```python
from build123d import *

# Parameters (mm, degrees)
SKETCH2_W             = 470
SKETCH2_H             = 317
BOSS_EXTRUDE1_DEPTH   = 5
SKETCH3_R             = 4.05
CUT_EXTRUDE1_DEPTH    = 10
SKETCH4_R             = 9
CUT_EXTRUDE2_DEPTH    = 11
M5X0_8_TAPPED_HOLE1_D = 4.2
SKETCH7_R             = 19.1
CUT_EXTRUDE5_DEPTH    = 2
M5X0_8_TAPPED_HOLE2_D = 4.2
SKETCH19_R            = 15
CUT_EXTRUDE10_DEPTH   = 9
SKETCH20_W            = 14
SKETCH20_H            = 30
CUT_EXTRUDE11_DEPTH   = 2
M3X0_5_TAPPED_HOLE2_D = 2.5
SKETCH23_W            = 14
SKETCH23_H            = 13.5
CUT_EXTRUDE13_DEPTH   = 9
CUT_EXTRUDE14_DEPTH   = 11
FILLET1_R             = 3
FILLET2_R             = 2.5
SKETCH27_R            = 4.05
CUT_EXTRUDE15_DEPTH   = 11
CUT_EXTRUDE16_DEPTH   = 11
CUT_EXTRUDE17_DEPTH   = 11


with BuildPart() as part:
    # Sketch2 → Boss-Extrude1 (new body, symmetric)
    with BuildSketch(Plane.XY):
        Rectangle(SKETCH2_W, SKETCH2_H)
    extrude(amount=BOSS_EXTRUDE1_DEPTH, both=True)

    # Sketch3 → Cut-Extrude1 (cut)
    with BuildSketch(Plane.XY.offset(5)):
        with Locations((-215, -83.5)):
            Circle(SKETCH3_R)
        with Locations((-215, -143.5)):
            Circle(SKETCH3_R)
        with Locations((215, -143.5)):
            Circle(SKETCH3_R)
        with Locations((-62.5, 133.34)):
            Circle(SKETCH3_R)
        with Locations((215, 138.5)):
            Circle(SKETCH3_R)
    extrude(amount=-CUT_EXTRUDE1_DEPTH, mode=Mode.SUBTRACT)

    # Sketch4 → Cut-Extrude2 (cut, through all)
    with BuildSketch(Plane.XY.offset(5)):
        with Locations((112.65, 121)):
            Circle(SKETCH4_R)
        with Locations((112.65, 26.5)):
            Circle(SKETCH4_R)
    extrude(amount=-CUT_EXTRUDE2_DEPTH, mode=Mode.SUBTRACT)

    # M5x0.8 Tapped Hole1 (through all)
    with Locations(Plane.XY.offset(5)):
        with Locations((132.65, 121), (92.65, 121), (92.65, 26.5), (132.65, 26.5)):
            Hole(M5X0_8_TAPPED_HOLE1_D / 2)

    # Sketch7 → Cut-Extrude5 (cut)
    with BuildSketch(Plane.XY.offset(5)):
        with Locations((112.05, 73.75)):
            Circle(SKETCH7_R)
    extrude(amount=-CUT_EXTRUDE5_DEPTH, mode=Mode.SUBTRACT)

    # M5x0.8 Tapped Hole2 (through all)
    with Locations(Plane.XY.offset(5)):
        with Locations((88.45, 97.35), (135.65, 97.35), (135.65, 50.15), (88.45, 50.15)):
            Hole(M5X0_8_TAPPED_HOLE2_D / 2)

    # Sketch19 → Cut-Extrude10 (cut, through all)
    with BuildSketch(Plane.XY.offset(3)):
        with Locations((112.05, 73.75)):
            Circle(SKETCH19_R)
    extrude(amount=-CUT_EXTRUDE10_DEPTH, mode=Mode.SUBTRACT)

    # Sketch20 → Cut-Extrude11 (cut)
    with BuildSketch(Plane.XY.offset(5)):
        with Locations((84.65, -3.5)):
            Rectangle(SKETCH20_W, SKETCH20_H)
    extrude(amount=-CUT_EXTRUDE11_DEPTH, mode=Mode.SUBTRACT)

    # M3x0.5 Tapped Hole2 (through all)
    with Locations(Plane.XY.offset(3)):
        with Locations((83.65, 6.5), (83.65, -13.5)):
            Hole(M3X0_5_TAPPED_HOLE2_D / 2)

    # Sketch23 → Cut-Extrude13 (cut, through all)
    with BuildSketch(Plane.XY.offset(3)):
        with Locations((84.65, -3.5)):
            Rectangle(SKETCH23_W, SKETCH23_H)
    extrude(amount=-CUT_EXTRUDE13_DEPTH, mode=Mode.SUBTRACT)

    # Sketch26 → Cut-Extrude14 (cut, through all)
    with BuildSketch(Plane.XY.offset(5)):
        Polygon((-32.351626406, 191.772644842), (-286.046542749, -61.922271502), (-286.046542749, 282.491923936), align=None)
    extrude(amount=-CUT_EXTRUDE14_DEPTH, mode=Mode.SUBTRACT)

    # Fillet1
    fillet1_edges = [part.edges().sort_by_distance(p)[0] for p in [
        (77.65, 11.5, 4),
        (91.65, 3.25, -1),
        (91.65, -10.25, -1),
        (77.65, -10.25, -1),
        (77.65, 3.25, -1),
        (91.65, 11.5, 4),
        (91.65, -18.5, 4),
        (77.65, -18.5, 4),
    ]]
    fillet(fillet1_edges, radius=FILLET1_R)

    # Fillet2
    fillet2_edges = [part.edges().sort_by_distance(p)[0] for p in [
        (-65.624271247, 158.5, 0),
        (-235, -10.875728753, 0),
        (235, -158.5, 0),
        (-235, -158.5, 0),
        (235, 158.5, 0),
    ]]
    fillet(fillet2_edges, radius=FILLET2_R)

    # Sketch27 → Cut-Extrude15 (cut, through all)
    with BuildSketch(Plane.XY.offset(5)):
        with Locations((215, -83.5)):
            Circle(SKETCH27_R)
    extrude(amount=-CUT_EXTRUDE15_DEPTH, mode=Mode.SUBTRACT)

    # Sketch28 → Cut-Extrude16 (cut, through all)
    with BuildSketch(Plane.XY.offset(5)):
        with BuildLine():
            Line((-61.439339828, 123.086951673), (-57.550252532, 119.197864376))
            ThreePointArc((-57.550252532, 119.197864376), (-57.196699141, 119.051417767), (-56.843145751, 119.197864376))
            Line((-56.843145751, 119.197864376), (-48.357864376, 127.683145751))
            ThreePointArc((-48.357864376, 127.683145751), (-48.211417767, 128.036699141), (-48.357864376, 128.390252532))
            Line((-48.357864376, 128.390252532), (-52.246951673, 132.279339828))
            ThreePointArc((-52.246951673, 132.279339828), (-52.600505063, 132.425786438), (-52.954058454, 132.279339828))
            Line((-52.954058454, 132.279339828), (-61.439339828, 123.794058454))
            ThreePointArc((-61.439339828, 123.794058454), (-61.585786438, 123.440505063), (-61.439339828, 123.086951673))
        make_face()
    extrude(amount=-CUT_EXTRUDE16_DEPTH, mode=Mode.SUBTRACT)

    # Sketch29 → Cut-Extrude17 (cut, through all)
    with BuildSketch(Plane.XY.offset(5)):
        with BuildLine():
            Line((-207, -90), (-201.5, -90))
            ThreePointArc((-201.5, -90), (-201.146446609, -89.853553391), (-201, -89.5))
            Line((-201, -89.5), (-201, -77.5))
            ThreePointArc((-201, -77.5), (-201.146446609, -77.146446609), (-201.5, -77))
            Line((-201.5, -77), (-207, -77))
            ThreePointArc((-207, -77), (-207.353553391, -77.146446609), (-207.5, -77.5))
            Line((-207.5, -77.5), (-207.5, -89.5))
            ThreePointArc((-207.5, -89.5), (-207.353553391, -89.853553391), (-207, -90))
        make_face()
    extrude(amount=-CUT_EXTRUDE17_DEPTH, mode=Mode.SUBTRACT)


solid = part.part
```
Could you check a few things on this model? Use its own coordinates, in mm. A direction names the side the tool comes from. Give positions to 0.01 mm unless a question says otherwise; leave off trailing zeros. Loops run counter-clockwise (first coordinate to the right, second up) from the corner with the lowest first, then second, coordinate; pieces in that order, holes last. Notation, with made-up numbers: (-13, 5) - (-1, 5) arc R29 ccw to (-1, 39) - close; hole circle Ø11 at (-6, 37). An arc over 180 degrees is marked (long way). Answer in a Markdown table with one row per item. Add a question column.
Q1. If we section it at C-C (x = -97.5): List the corners of the cut face in (y, z) for me, plus the area to 3 significant figures.
Q2. Please list where these lines run through material, in increasing order: L1, parallel to Y at x = 112.65, z = 0.5; L2, parallel to Y at x = 135.65, z = -0.25; L3, parallel to Y at x = 111.5, z = -0.5. Write a range as from..to.
Q3. If we section it at A-A (x = 112.65): List the corners of the cut face in (y, z) for me, plus the area to 3 significant figures.
Q4. We'd pull the mould along Y, two halves only. Please class faces 4 (the face through (-235, -85, 0)), 5 (the face through (82, 158.5, 0)), 6 (the face through (91.65, -4, 1)): +Y half, -Y half, draft (parallel to the pull), parting line (faces both ways), or undercut.
Q5. If we section it at B-B (z = -0.5): State how many separate pieces and enclosed holes the cut face has, plus the area to 3 significant figures.
Q6. For pin 1 (6.5 mm diameter, centred on x = 88.45, y = 97.35, fed in from +Z); pin 2 (6 mm diameter, centred on x = -205, z = -0.5, fed in from +Y); pin 3 (4 mm diameter, centred on x = -115, z = -1, fed in from +Y); pin 4 (6 mm diameter, centred on x = -126, z = -3, fed in from +Y), each with a flat end and sliding along its axis, tell me the tip position at first contact or that it passes through.
Q7. Which directions (+Z, -Z, +X, -X, +Y, -Y) give clear straight access to the entire face, cutting with the end or side of a thin tool? Please do faces 1 (the face through (120.4, 61.1, 3)), 2 (the face through (-207.5, -83, 0)), 3 (the face through (-149.137, 74.988, 0.07)).
The answers:
| question | item | result |
|---|---|---|
| 1 | outline | (-158.5, -5) - (126.62, -5) - (126.62, 5) - (-158.5, 5) - close |
| 1 | area | 2,850 mm^2 |
| 2 | L1 | y = -158.5..17.5, 35.5..58.76, 88.74..112, 130..158.5 |
| 2 | L2 | y = -158.5..48.05, 52.25..95.25, 99.45..158.5 |
| 2 | L3 | y = -158.5..17.57, 35.43..58.76, 88.74..112.07, 129.93..158.5 |
| 3 | outline | (-158.5, -5) - (17.5, -5) - (17.5, 5) - (-158.5, 5) - close; (35.5, -5) - (58.76, -5) - (58.76, 3) - (54.66, 3) - (54.66, 5) - (35.5, 5) - close; (88.74, -5) - (112, -5) - (112, 5) - (92.84, 5) - (92.84, 3) - (88.74, 3) - close; (130, -5) - (158.5, -5) - (158.5, 5) - (130, 5) - close |
| 3 | area | 2,490 mm^2 |
| 4 | face 4 | draft |
| 4 | face 5 | +Y half |
| 4 | face 6 | undercut |
| 5 | separate pieces | 1 |
| 5 | enclosed holes | 22 |
| 5 | area | 133,000 mm^2 |
| 6 | pin 1 | stops at z = 5 |
| 6 | pin 2 | stops at y = 22.12 |
| 6 | pin 3 | stops at y = 111.12 |
| 6 | pin 4 | stops at y = 101.12 |
| 7 | face 1 | +Z |
| 7 | face 2 | +Z, -Z |
| 7 | face 3 | +Z, -Z, -X, +Y |
